Check sheet for the modelled part. Datum: model origin and axes. Units: mm. A direction names the side the tool comes from. Coordinates: 2 decimals unless noted, no trailing zeros. Loops run counter-clockwise (first coordinate to the right, second up) from the corner with the lowest first, then second, coordinate; pieces in that order, holes last.
```python
from build123d import *

# Parameters (mm, degrees)
BOSS_EXTRUDE1_DEPTH = 3.1877
SKETCH2_W           = 15.3289
SKETCH2_H           = 1.524
BOSS_EXTRUDE2_DEPTH = 2.0828
SKETCH3_R           = 3.30835
CUT_EXTRUDE1_DEPTH  = 15.567215559
CUT_EXTRUDE2_DEPTH  = 3.175


with BuildPart() as part:
    # Sketch1 → Boss-Extrude1 (new, symmetric)
    with BuildSketch(Plane(origin=(0, 0, 0), x_dir=(0, 0, -1), z_dir=(1, 0, 0))):
        with BuildLine():
            Line((9.906, 0), (-9.906, 0))
            ThreePointArc((-9.906, 0), (-11.522446102, 0.669553898), (-12.192, 2.286))
            Line((-12.192, 2.286), (-12.192, 5.6007))
            ThreePointArc((-12.192, 5.6007), (-11.016011939, 7.360690509), (-8.939961582, 6.947738418))
            Line((-8.939961582, 6.947738418), (-5.572365536, 3.580142373))
            Line((-5.572365536, 3.580142373), (-6.649996271, 2.502511638))
            Line((-6.649996271, 2.502511638), (-10.017592316, 5.870107684))
            ThreePointArc((-10.017592316, 5.870107684), (-10.432802388, 5.952698102), (-10.668, 5.6007))
            Line((-10.668, 5.6007), (-10.668, 2.286))
            ThreePointArc((-10.668, 2.286), (-10.444815367, 1.747184633), (-9.906, 1.524))
            Line((-9.906, 1.524), (9.906, 1.524))
            ThreePointArc((9.906, 1.524), (10.444815367, 1.747184633), (10.668, 2.286))
            Line((10.668, 2.286), (10.668, 5.6007))
            ThreePointArc((10.668, 5.6007), (10.432802388, 5.952698102), (10.017592316, 5.870107684))
            Line((10.017592316, 5.870107684), (6.649996271, 2.502511638))
            Line((6.649996271, 2.502511638), (5.572365536, 3.580142373))
            Line((5.572365536, 3.580142373), (8.939961582, 6.947738418))
            ThreePointArc((8.939961582, 6.947738418), (11.016011939, 7.360690509), (12.192, 5.6007))
            Line((12.192, 5.6007), (12.192, 2.286))
            ThreePointArc((12.192, 2.286), (11.522446102, 0.669553898), (9.906, 0))
        make_face()
    extrude(amount=BOSS_EXTRUDE1_DEPTH, both=True)

    # Sketch2 → Boss-Extrude2 (add)
    with BuildSketch(Plane(origin=(3.1877, 0, 0), x_dir=(0, 0, -1), z_dir=(1, 0, 0))):
        with Locations((0, 0.762)):
            Rectangle(SKETCH2_W, SKETCH2_H)
    boss_extrude2 = extrude(amount=BOSS_EXTRUDE2_DEPTH)

    # Mirror1: Boss-Extrude2 across plane
    add(boss_extrude2.mirror(Plane(origin=(0, 0, 0), x_dir=(0, 0, 1), z_dir=(1, 0, 0))))

    # Sketch3 → Cut-Extrude1 (cut, through all)
    with BuildSketch(Plane(origin=(0, 1.524, 0), x_dir=(1, 0, 0), z_dir=(0, 1, 0))):
        with Locations(Location((0, 0, 0), (0, 0, 270))):
            Circle(SKETCH3_R)
    extrude(amount=-CUT_EXTRUDE1_DEPTH, mode=Mode.SUBTRACT)

    # Sketch4 → Revolve1 (revolve)
    with BuildSketch(Plane(origin=(0, 0, 0), x_dir=(0, 0, -1), z_dir=(1, 0, 0)), mode=Mode.PRIVATE) as revolve1_sk:
        with BuildLine():
            Line((3.175, 0), (5.2705, 0))
            Line((5.2705, 0), (5.2705, -0.7874))
            ThreePointArc((5.2705, -0.7874), (4.374468906, -2.11435755), (3.175, -3.175))
            Line((3.175, -3.175), (0, -3.175))
            Line((0, -3.175), (0, 12.7))
            Line((0, 12.7), (2.159, 12.7))
            Line((2.159, 12.7), (3.175, 11.684))
            Line((3.175, 11.684), (3.175, 0))
        make_face()
    revolve(revolve1_sk.sketch.rotate(Axis((0, 19.260698501, 0), (0, -1, 0)), 180), axis=Axis((0, 19.260698501, 0), (0, -1, 0)))

    # Sketch5 → Cut-Extrude2 (cut)
    with BuildSketch(Plane.XZ.offset(3.175)):
        Polygon((0, 2.287692707), (-1.9812, 1.143846353), (-1.9812, -1.143846353), (0, -2.287692707), (1.9812, -1.143846353), (1.9812, 1.143846353), align=None)
    extrude(amount=-CUT_EXTRUDE2_DEPTH, mode=Mode.SUBTRACT)


solid = part.part
```
1) Set-up check for faces 1 (the flat face through (0.04, 4.21, -8.36)), 2 (the cylindrical face through (2.8, 5.8, 1.5)), 3 (the flat face through (-1, -1.61, -1.71)), 4 (the flat face through (0.04, 5.24, -7.23)), 5 (the flat face through (-4, 1, -7.664)): record each of +Z, -Z, +X, -X, +Y, -Y from which the full face is reachable in a straight line by a thin tool's end or side.
Answer sheet:
face 1: +X, -X
face 2: +Y
face 3: -Y
face 4: +X, -X, +Y
face 5: -Z, -X, +Y, -Y
2) Section check A-A on z = 8.5. Enter the section's corners in (x, y), plus the area to 3 significant figures.
Answer sheet:
outline: (-3.19, 0) - (3.19, 0) - (3.19, 1.52) - (-3.19, 1.52) - close; (-3.19, 4.35) - (3.19, 4.35) - (3.19, 6.51) - (-3.19, 6.51) - close
area: 23.5 mm2
3) Section check B-B on y = 10. Enter the section's corners in (x, z) (3 decimals), plus the area to 3 significant figures.
Answer sheet:
outline: circle Ø6.35 at (0, 0)
area: 31.7 mm2
4) Depth check by flat-ended pin: pin 1 (1.2 mm diameter, centred on x = -4, y = 0.5, fed in from -Z); pin 2 (3 mm diameter, centred on x = -3.5, z = 5.5, fed in from -Y); pin 3 (2 mm diameter, centred on x = 0, z = 0, fed in from -Y). Enter the tip coordinate at first touch or a pass-through.
Answer sheet:
pin 1: stops at z = -7.66
pin 2: stops at y = -1.24
pin 3: stops at y = 0
5) Scan lines: line 1 (Z direction, x = -2, y = 0.5); line 2 (Y direction, x = 0.5, z = -8); line 3 (Z direction, x = -0.25, y = 6.75). Record each from-to range of solid material in increasing order.
Answer sheet:
line 1: z = -11.33 to -2.64, -2.47 to 2.47, 2.64 to 11.33
line 2: y = 0 to 1.52, 3.85 to 6.01
line 3: z = -11.81 to -8.74, -3.17 to 3.17, 8.74 to 11.81
6) Mould release check, pull along Z, two halves, no side actions. Record for faces 6 (the flat face through (0.04, 5.29, 7.28)), 7 (the flat face through (0, 0, 6)), 8 (the flat face through (0, 4, -12.192)): +Z half, -Z half, draft (parallel to the pull), parting line (faces both ways), or undercut.
Answer sheet:
face 6: undercut
face 7: draft
face 8: -Z half
